Here's the drawing with two shaded views (mm, measured from the low corner). I have some questions. A direction names the side the tool comes from. Give positions to 0.01 mm unless a question says otherwise; leave off trailing zeros. Order: outer loops, then holes, each group sorted by start corner. A loop starts at its lowest first (then second) coordinate and runs counter-clockwise, first axis right, second up. Notation, with made-up numbers: M 7,-7.5 L 14,-7.5 A25 ccw 14,15.5 Z; hole C 83,33 d11. An arc over 180 degrees is marked long. Write each question's results on one line, items separated by ' | '.
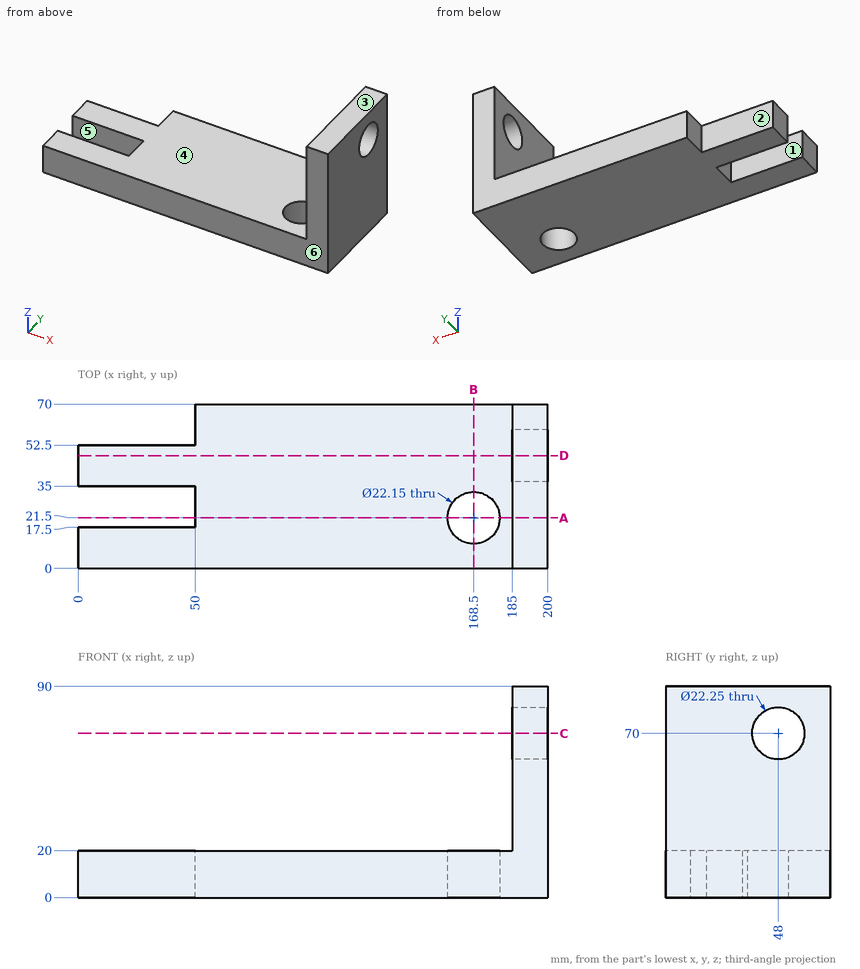
(1) Imagine slicing it at B-B, the plane x = 168.5. Write out the boundary of the cut face in (y, z) (3 decimals).
Data:
outline: M 0,0 L 10.425,0 L 10.425,20 L 0,20 Z; M 32.575,0 L 70,0 L 70,20 L 32.575,20 Z
(2) Imagine slicing it at D-D, the plane y = 48. Write out the boundary of the cut face in (x, z) (3 decimals).
Data:
outline: M 0,0 L 200,0 L 200,58.875 L 185,58.875 L 185,20 L 0,20 Z; M 185,81.125 L 200,81.125 L 200,90 L 185,90 Z
(3) We'd pull the mould along Y, two halves only. Please class the marked faces 1, 2 and 3: +Y half, -Y half, draft (parallel to the pull), parting line (faces both ways), or undercut.
Data:
face 1: undercut | face 2: +Y half | face 3: draft
(4) Will these pins go through, and if not, where does the flat tip stop? P1, Ø16, axis at x = 12.5, z = 6.5, coming from the +Y side; P2, Ø5, axis at x = 148, y = 48, coming from the +Z side; P3, Ø5, axis at y = 27.5, z = 32, coming from the -X side; P4, Ø20, axis at x = 168.5, y = 21.5, coming from the +Z side.
Data:
P1: stops at y = 52.5 | P2: stops at z = 20 | P3: stops at x = 185 | P4: passes through
(5) I need wall thicknesses on L1, parallel to Y at x = 48, z = 5; L2, parallel to Y at x = 168.5, z = 7.75 (3 decimals); L3, parallel to X at y = 6, z = 52. Which ranges of each line are inside material? Lowest first, please. Write a range as from..to.
Data:
L1: y = 0..17.5, 35..52.5 | L2: y = 0..10.425, 32.575..70 | L3: x = 185..200
(6) Imagine slicing it at A-A, the plane y = 21.5. Write out the boundary of the cut face in (x, z) (3 decimals), plus the area to 3 significant figures.
Data:
outline: M 50,0 L 157.425,0 L 157.425,20 L 50,20 Z; M 179.575,0 L 200,0 L 200,90 L 185,90 L 185,20 L 179.575,20 Z | area: 3,610 mm2
(7) Imagine slicing it at C-C, the plane z = 70. Write out the boundary of the cut face in (x, y) (3 decimals).
Data:
outline: M 185,0 L 200,0 L 200,36.875 L 185,36.875 Z; M 185,59.125 L 200,59.125 L 200,70 L 185,70 Z
(8) For the marked faces 4, 5 and 6, which set-ups out of +Z, -Z, +X, -X, +Y, -Y let a thin tool reach every point of the face, with its end or its side?
Data:
face 4: +Z, -X, +Y, -Y | face 5: +Z, -Z, -X | face 6: +Z, -Z, +X, -X, -Y
